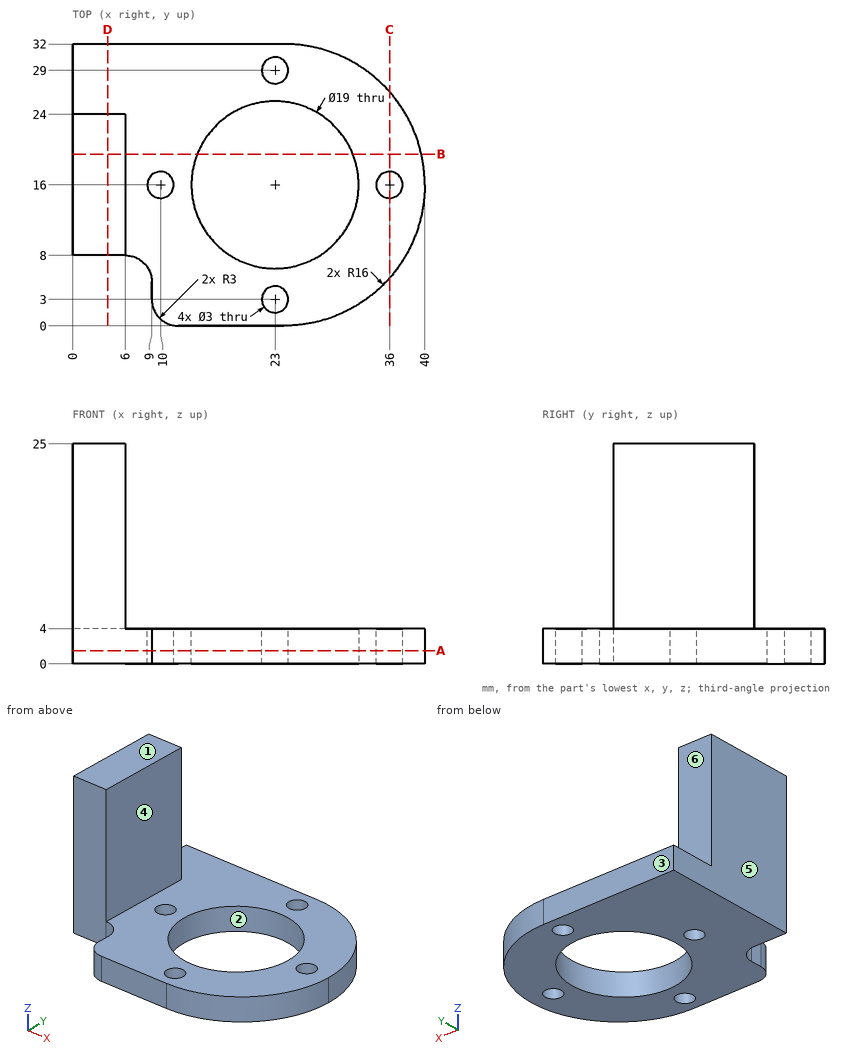
Here's the drawing with two shaded views (mm, measured from the low corner). I have some questions. A direction names the side the tool comes from. Coordinates: 2 decimals unless noted, no trailing zeros. Write each loop counter-clockwise with the first axis right and the second up, starting at its lowest first coordinate (ties: lowest second). Pieces come first, ordered by that corner, then holes.
Item 1: If we mould it in two halves opening along Y, with no side actions, what happens to the marked faces 1, 2 and 3? For each: +Y half, -Y half, draft (parallel to the pull), parting line (faces both ways), or undercut.
Item 2: If I drill on line 1 (Y direction, x = 23, z = 1.7); line 2 (Z direction, x = 15.5, y = 22); line 3 (X direction, y = 11.5, z = 5.5), over which ranges is the centre line in solid material (lowest first)?
Item 3: I want a section at C-C on x = 36. Write out the boundary of the cut face in (y, z).
Item 4: I want a section at B-B on y = 19.5. Write out the boundary of the cut face in (x, z).
Item 5: I want a section at A-A on z = 1.5. Count the separate pieces of the cut face and the enclosed holes in it, and give its area (3 significant figures).
Item 6: On a 3-axis mill with a long thin cutter (end or side, diameter ignored), from which of +Z, -Z, +X, -X, +Y, -Y can I reach the whole of each face in a straight line? I mean the marked faces 4, 5 and 6. Say none if no direction works.
Item 7: Will these pins go through, and if not, where does the flat tip stop? pin 1 (10 mm diameter, centred on y = 21.5, z = 10, fed in from +X); pin 2 (5 mm diameter, centred on x = 18, y = 21.5, fed in from +Z); pin 3 (15 mm diameter, centred on x = 23, y = 16, fed in from -Z); pin 4 (2 mm diameter, centred on y = 4, z = 2, fed in from -X).
Item 8: I want a section at D-D on x = 4. Write out the boundary of the cut face in (y, z).
Findings below:
1. face 1: draft
1. face 2: undercut
1. face 3: +Y half
2. line 1: y = 0 to 1.5, 4.5 to 6.5, 25.5 to 27.5, 30.5 to 32
2. line 2: z = 0 to 4
2. line 3: x = 0 to 6
3. outline: (5.42, 0) - (14.5, 0) - (14.5, 4) - (5.42, 4) - close; (17.5, 0) - (26.58, 0) - (26.58, 4) - (17.5, 4) - close
4. outline: (0, 0) - (14.17, 0) - (14.17, 4) - (6, 4) - (6, 25) - (0, 25) - close; (31.83, 0) - (39.61, 0) - (39.61, 4) - (31.83, 4) - close
5. separate pieces: 1
5. enclosed holes: 5
5. area: 786 mm2
6. face 4: +Z, +X, +Y, -Y
6. face 5: +Z, -Z, -X, +Y, -Y
6. face 6: +Z, +X, -X, +Y
7. pin 1: stops at x = 6
7. pin 2: stops at z = 4
7. pin 3: passes through
7. pin 4: stops at x = 9
8. outline: (8, 0) - (32, 0) - (32, 4) - (24, 4) - (24, 25) - (8, 25) - close
